CAD build for the part. Positions are in the model's coordinates, mm. A direction names the side the tool comes from. Round coordinates to 2 decimals unless told otherwise and drop trailing zeros. Order: outer loops, then holes, each group sorted by start corner. A loop starts at its lowest first (then second) coordinate and runs counter-clockwise, first axis right, second up. Notation, with made-up numbers: (20, -39) - (24, -39) arc R15 ccw to (24, -24) - close; hole circle Ø6 at (-31, 29.5). An arc over 180 degrees is marked (long way). Use one line per item in the form item = value. Start each with the question number.
from build123d import *

# Parameters (mm, degrees)
BOSS_EXTRUDE1_DEPTH     = 45
CUT_EXTRUDE1_REACH      = 22
SKETCH3_R               = 1.2
CUT_EXTRUDE2_DEPTH      = 10
CUT_EXTRUDE3_DEPTH      = 1
CUT_EXTRUDE3_DEPTH_BACK = 51


with BuildPart() as part:
    # Sketch1 → Boss-Extrude1 (new body)
    with BuildSketch(Plane.XY):
        Polygon((-25, 0), (-20, 0), (-20, 15), (20, 15), (20, 0), (25, 0), (25, 20), (-25, 20), align=None)
    extrude(amount=BOSS_EXTRUDE1_DEPTH)

    # Sketch2 → Cut-Extrude1 (cut, up to next)
    with BuildSketch(Plane(origin=(0, 20, 0), x_dir=(1, 0, 0), z_dir=(0, 1, 0)), mode=Mode.PRIVATE) as cut_extrude1_sk1:
        with BuildLine():
            Line((11.25, 0), (11.25, -22.5))
            ThreePointArc((11.25, -22.5), (0, -33.75), (-11.25, -22.5))
            Line((-11.25, -22.5), (-11.25, 0))
            Line((-11.25, 0), (11.25, 0))
        make_face()
    cut_extrude1_tool1 = extrude(cut_extrude1_sk1.sketch, amount=-CUT_EXTRUDE1_REACH, mode=Mode.PRIVATE) & part.part
    add(cut_extrude1_tool1.solids().sort_by_distance((0, 20, 15.768467))[0], mode=Mode.SUBTRACT)

    # Sketch3 → Cut-Extrude2 (cut)
    with BuildSketch(Plane(origin=(0, 20, 0), x_dir=(1, 0, 0), z_dir=(0, 1, 0))):
        with Locations((15.85, -36)):
            Circle(SKETCH3_R)
        with Locations((-14.15, -36)):
            Circle(SKETCH3_R)
        with Locations((-14.15, -5)):
            Circle(SKETCH3_R)
        with Locations((15.85, -5)):
            Circle(SKETCH3_R)
    extrude(amount=-CUT_EXTRUDE2_DEPTH, mode=Mode.SUBTRACT)

    # Sketch4 → Cut-Extrude3 (cut, two sides)
    with BuildSketch(Plane(origin=(25, 0, 0), x_dir=(0, 0, -1), z_dir=(1, 0, 0))) as cut_extrude3_sk:
        with BuildLine():
            Line((-35.9, 11.6), (-35.9, 4.1))
            ThreePointArc((-35.9, 4.1), (-37.5, 2.5), (-39.1, 4.1))
            Line((-39.1, 4.1), (-39.1, 11.6))
            ThreePointArc((-39.1, 11.6), (-37.5, 13.2), (-35.9, 11.6))
        make_face()
        with BuildLine():
            Line((-9.1, 11.6), (-9.1, 4.1))
            ThreePointArc((-9.1, 4.1), (-7.5, 2.5), (-5.9, 4.1))
            Line((-5.9, 4.1), (-5.9, 11.6))
            ThreePointArc((-5.9, 11.6), (-7.5, 13.2), (-9.1, 11.6))
        make_face()
    extrude(amount=CUT_EXTRUDE3_DEPTH, mode=Mode.SUBTRACT)
    extrude(cut_extrude3_sk.sketch, amount=-CUT_EXTRUDE3_DEPTH_BACK, mode=Mode.SUBTRACT)


solid = part.part
(1) Slice it at C-C (z = 7.5). Give the cut face in (x, y).
(2) Which spindle directions (+Z, -Z, +X, -X, +Y, -Y) get a long thin tool onto all of the face, cutting with end or side? Do faces 3 (the flat face through (11.25, 18, 11)), 4 (the flat face through (-20, 7, 22)), 5 (the cylindrical face through (14.65, 17.54, 4.95)), 6 (the flat face through (23, 8, 9.1)), 7 (the flat face through (11, 20, 27)). Say none if no direction does.
(3) Wall check: line 1 (Z direction, x = 15.85, y = 18.5); line 2 (X direction, y = 18.2, z = 5); line 3 (X direction, y = 16.05, z = 36). Give the ranges that are in metal, low to high. Write a range as [from, to].
(4) Slice it at A-A (x = 15.85). Give the cut face in (y, z), and give its area (3 significant figures).
(5) Slice it at B-B (y = 14). Give the cut face in (x, z).
(6) Mould opens along X. For faces 1 (the cylindrical face through (-13.005, 17.535, 4.64)), 2 (the cylindrical face through (22.5, 13.2, 7.5)) say: pulls with the +X half, pulls with the -X half, needs draft (parallel to the pull), parting line crosses it, or undercut.
(7) Flat gauge pin, fed straight in: P1, Ø12, axis at x = -10, z = 15.5, coming from the -Y side. Where does the tip first touch, or does it go through?
(8) Slice it at D-D (z = 14). Give the cut face in (x, y).
Results list:
q1.outline = (-25, 0) - (-20, 0) - (-20, 2.5) - (-25, 2.5) - close; (-25, 13.2) - (-20, 13.2) - (-20, 15) - (-11.25, 15) - (-11.25, 20) - (-25, 20) - close; (11.25, 15) - (20, 15) - (20, 13.2) - (25, 13.2) - (25, 20) - (11.25, 20) - close; (20, 0) - (25, 0) - (25, 2.5) - (20, 2.5) - close
q2.face_3 = -Z, +Y, -Y
q2.face_4 = +Z, -Z, -Y
q2.face_5 = +Y, -Y
q2.face_6 = +X, -X
q2.face_7 = +Z, -Z, +X, -X, +Y
q3.line_1 = [0, 3.8], [6.2, 34.8], [37.2, 45]
q3.line_2 = [-25, -15.35], [-12.95, -11.25], [11.25, 14.65], [17.05, 25]
q3.line_3 = [-25, -15.35], [-12.95, 14.65], [17.05, 25]
q4.outline = (15, 0) - (20, 0) - (20, 3.8) - (15, 3.8) - close; (15, 6.2) - (20, 6.2) - (20, 34.8) - (15, 34.8) - close; (15, 37.2) - (20, 37.2) - (20, 45) - (15, 45) - close
q4.area = 201 mm²
q5.outline = (-25, 0) - (-20, 0) - (-20, 45) - (-25, 45) - close; (20, 0) - (25, 0) - (25, 45) - (20, 45) - close
q6.face_1 = undercut
q6.face_2 = needs draft
q7.P1 = 15
q8.outline = (-25, 0) - (-20, 0) - (-20, 15) - (-11.25, 15) - (-11.25, 20) - (-25, 20) - close; (11.25, 15) - (20, 15) - (20, 0) - (25, 0) - (25, 20) - (11.25, 20) - close
